```python
from build123d import *
from build123d import SkipClean  # not in build123d's __all__

# Parameters (mm, degrees)
F0_W     = 9
F0_H     = 9
F1_DEPTH = 3
F2_DEPTH = 20
F3_DEPTH = 25
F4_R     = 2


with BuildPart() as f1:
    # F0 (on Top) → F1 (new body)
    with BuildSketch(Plane.XY):
        with BuildLine():
            ThreePointArc((17, -10.5356537529), (19.2353840617, -5.4772255751), (20, 0))
            ThreePointArc((20, 0), (19.2353840617, 5.4772255751), (17, 10.5356537529))
            add(Edge.make_bspline(
                [(17, -10.5356537529), (15.4390588775, -5.7747014672), (13.767943494, 0), (15.4390588775, 5.7747014672), (17, 10.5356537529)],
                knots=[0, 0, 0, 0, 0.5, 1, 1, 1, 1], degree=3))
        make_face()
        with BuildLine():
            add(Edge.make_bspline(
                [(17, -10.5356537529), (15.4390588775, -5.7747014672), (13.767943494, 0), (15.4390588775, 5.7747014672), (17, 10.5356537529)],
                knots=[0, 0, 0, 0, 0.5, 1, 1, 1, 1], degree=3))
            ThreePointArc((17, 10.5356537529), (0, 20), (-17, 10.5356537529))
            add(Edge.make_bspline(
                [(-17, -10.5356537529), (-15.4390588775, -5.7747014672), (-13.767943494, 0), (-15.4390588775, 5.7747014672), (-17, 10.5356537529)],
                knots=[0, 0, 0, 0, 0.5, 1, 1, 1, 1], degree=3))
            ThreePointArc((-17, -10.5356537529), (0, -20), (17, -10.5356537529))
        make_face()
        Rectangle(F0_W, F0_H, mode=Mode.SUBTRACT)
        with BuildLine():
            add(Edge.make_bspline(
                [(-17, -10.5356537529), (-15.4390588775, -5.7747014672), (-13.767943494, 0), (-15.4390588775, 5.7747014672), (-17, 10.5356537529)],
                knots=[0, 0, 0, 0, 0.5, 1, 1, 1, 1], degree=3))
            ThreePointArc((-17, 10.5356537529), (-20, 0), (-17, -10.5356537529))
        make_face()
        Rectangle(F0_W, F0_H)
    extrude(amount=F1_DEPTH)

    # F0 (on Top) → F2 (join)
    with BuildSketch(Plane.XY):
        with BuildLine():
            add(Edge.make_bspline(
                [(17, -10.5356537529), (15.4390588775, -5.7747014672), (13.767943494, 0), (15.4390588775, 5.7747014672), (17, 10.5356537529)],
                knots=[0, 0, 0, 0, 0.5, 1, 1, 1, 1], degree=3))
            ThreePointArc((17, 10.5356537529), (0, 20), (-17, 10.5356537529))
            add(Edge.make_bspline(
                [(-17, -10.5356537529), (-15.4390588775, -5.7747014672), (-13.767943494, 0), (-15.4390588775, 5.7747014672), (-17, 10.5356537529)],
                knots=[0, 0, 0, 0, 0.5, 1, 1, 1, 1], degree=3))
            ThreePointArc((-17, -10.5356537529), (0, -20), (17, -10.5356537529))
        make_face()
        Rectangle(F0_W, F0_H, mode=Mode.SUBTRACT)
    with SkipClean():  # cleaning this boolean's faces spoils the solid; the shape is the same uncleaned
        extrude(amount=F2_DEPTH)

    # F0 (on Top) → F3 (cut)
    with BuildSketch(Plane.XY):
        with BuildLine():
            add(Edge.make_bspline(
                [(-17, -10.5356537529), (-15.4390588775, -5.7747014672), (-13.767943494, 0), (-15.4390588775, 5.7747014672), (-17, 10.5356537529)],
                knots=[0, 0, 0, 0, 0.5, 1, 1, 1, 1], degree=3))
            ThreePointArc((-17, 10.5356537529), (-20, 0), (-17, -10.5356537529))
        make_face()
        with BuildLine():
            ThreePointArc((17, -10.5356537529), (19.2353840617, -5.4772255751), (20, 0))
            ThreePointArc((20, 0), (19.2353840617, 5.4772255751), (17, 10.5356537529))
            add(Edge.make_bspline(
                [(17, -10.5356537529), (15.4390588775, -5.7747014672), (13.767943494, 0), (15.4390588775, 5.7747014672), (17, 10.5356537529)],
                knots=[0, 0, 0, 0, 0.5, 1, 1, 1, 1], degree=3))
        make_face()
    extrude(amount=F3_DEPTH, mode=Mode.SUBTRACT)

    # F4
    f4_edges = [f1.edges().sort_by_distance(p)[0] for p in [
        (0, 20, 0),
        (-14.603501, 0, 0),
        (0, -20, 0),
        (14.603501, 0, 0),
        (-17, 10.535654, 1.5),
        (-17, 10.535654, 11.5),
        (-17, -10.535654, 1.5),
        (-17, -10.535654, 11.5),
        (17, 10.535654, 1.5),
        (17, 10.535654, 11.5),
        (17, -10.535654, 11.5),
        (17, -10.535654, 1.5),
    ]]
    fillet(f4_edges, radius=F4_R)


solid = f1.part
```
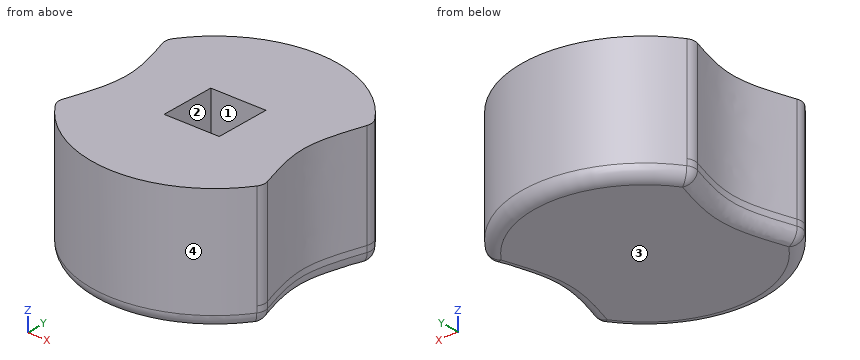
Input: part model. Units: mm. Frame: model coordinates. Face numbers are marked on the shaded views. Round coordinates to 2 decimals unless told otherwise and drop trailing zeros. Write each loop counter-clockwise with the first axis right and the second up, starting at its lowest first coordinate (ties: lowest second). Pieces come first, ordered by that corner, then holes. Notation, with made-up numbers: (-28.5, -8.75) -> (20.5, -8.75) arc R7 cw to (20.5, 2.25) -> close; hole circle Ø1 at (44.5, -17.75). An arc over 180 degrees is marked (long way). Answer as CSV lines item,"result".
1. Ray query, L1, parallel to X at y = 0.5, z = 13; L2, parallel to X at y = 2.5, z = 18; L3, parallel to Y at x = 0, z = 18. Return the intervals inside material, ascending. Write a range as [from, to].
Geometry says:
L1,"x = [-14.61, -4.5], [4.5, 14.61]"
L2,"x = [-14.8, -4.5], [4.5, 14.8]"
L3,"y = [-20, -4.5], [4.5, 20]"
2. Section A-A (x = 0). Return the cut outline in (y, z).
Geometry says:
outline,"(-20, 2) arc R2 ccw to (-18, 0) -> (18, 0) arc R2 ccw to (20, 2) -> (20, 20) -> (4.5, 20) -> (4.5, 3) -> (-4.5, 3) -> (-4.5, 20) -> (-20, 20) -> close"
3. Mould query, pull axis X, two halves, no side actions, for the marked faces 1, 2, 3 and 4. Classes: +X half, -X half, draft (parallel to the pull), parting line (faces both ways), or undercut.
Geometry says:
face 1,"undercut"
face 2,"undercut"
face 3,"draft"
face 4,"parting line"
4. Contact query for flat-ended pins moving along their axis: P1, Ø2.5, axis at y = -1.5, z = 13, coming from the -X side; P2, Ø4.5, axis at y = -0.5, z = 8.5, coming from the +X side; P3, Ø4, axis at x = 5.5, z = 16.5, coming from the +Y side. Output: stop coordinate, or through.
Geometry says:
P1,"stops at x = -14.84"
P2,"stops at x = 14.84"
P3,"stops at y = 19.69"
